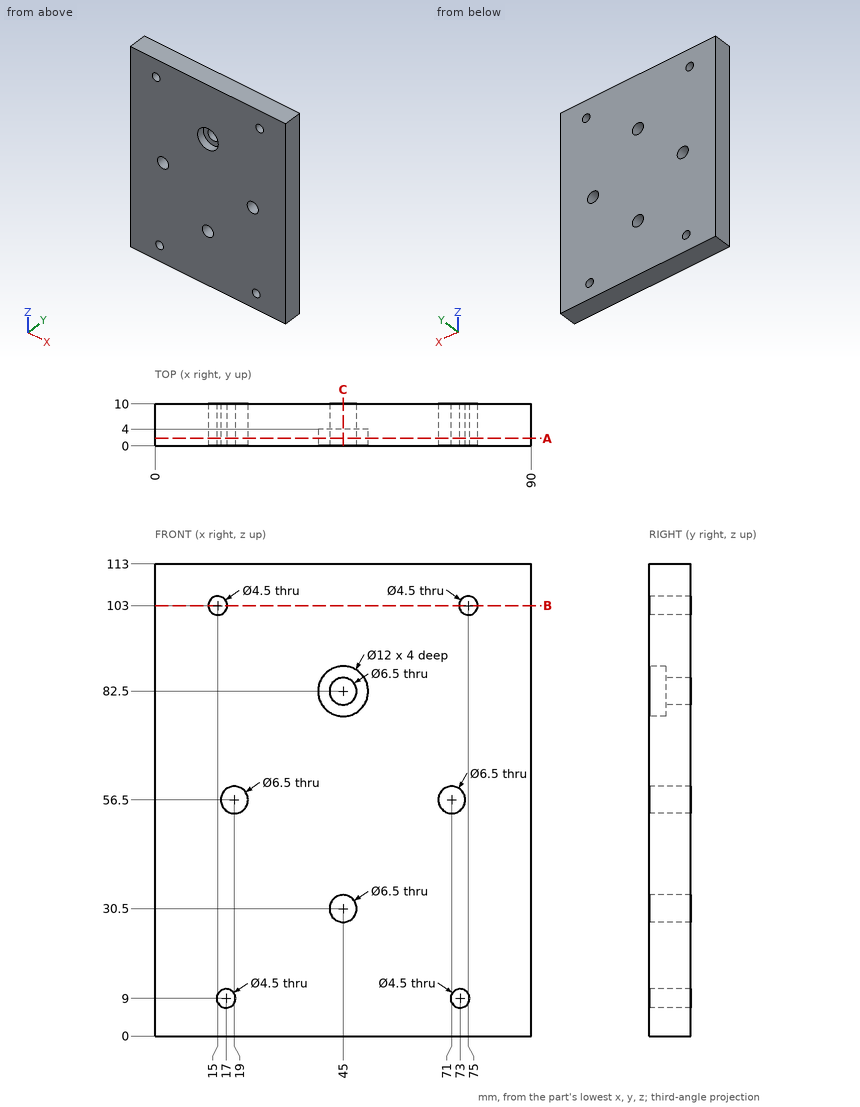
Geometry: see drawing. Coordinates: mm, zero at the bounding-box minimum. Coordinates: 2 decimals unless noted, no trailing zeros. Order: outer loops, then holes, each group sorted by start corner. A loop starts at its lowest first (then second) coordinate and runs counter-clockwise, first axis right, second up. Notation, with made-up numbers: M 4,64.25 L 21,64.25 A29 cw 21,88.25 Z; hole C -4,-1 d4. An arc over 180 degrees is marked long. Write item = value, one per line. Start each with the question number.
(1) Section A-A on y = 1.75. Give the number of separate pieces and of enclosed holes in the cut face, and give its area (3 significant figures).
(2) Section C-C on x = 45. Output: boundary loops of the cut face in (y, z), and give its area (3 significant figures).
(3) First-contact query: P1, Ø7.5, axis at x = 71, z = 56.5, coming from the +Y side; P2, Ø3.5, axis at x = 47, z = 84, coming from the -Y side. Flat tips, straight axial feed; report the tip coordinate or a pass-through.
(4) Line query: line 1 along Z through (x, y) = (45, 3.25); line 2 along Z through (x, y) = (71, 3); line 3 along X through (y, z) = (4.25, 102.5). Output: solid intervals per line, ascending. Write a range as [from, to].
(5) Section B-B on z = 103. Output: boundary loops of the cut face in (x, y), and give its area (3 significant figures).
Result set:
q1.separate_pieces = 1
q1.enclosed_holes = 8
q1.area = 9,890 mm²
q2.outline = M 0,0 L 10,0 L 10,27.25 L 0,27.25 Z; M 0,33.75 L 10,33.75 L 10,79.25 L 4,79.25 L 4,76.5 L 0,76.5 Z; M 0,88.5 L 4,88.5 L 4,85.75 L 10,85.75 L 10,113 L 0,113 Z
q2.area = 978 mm²
q3.P1 = 10
q3.P2 = 4
q4.line_1 = [0, 27.25], [33.75, 76.5], [88.5, 113]
q4.line_2 = [0, 7.97], [10.03, 53.25], [59.75, 113]
q4.line_3 = [0, 12.81], [17.19, 72.81], [77.19, 90]
q5.outline = M 0,0 L 12.75,0 L 12.75,10 L 0,10 Z; M 17.25,0 L 72.75,0 L 72.75,10 L 17.25,10 Z; M 77.25,0 L 90,0 L 90,10 L 77.25,10 Z
q5.area = 810 mm²
